Source: three-view drawing plus pictorial views. Frame: mm from the lowest corner of the part. A direction names the side the tool comes from. Give positions to 0.01 mm unless a question says otherwise; leave off trailing zeros. Write each loop counter-clockwise with the first axis right and the second up, starting at its lowest first coordinate (ties: lowest second). Pieces come first, ordered by that corner, then holes.
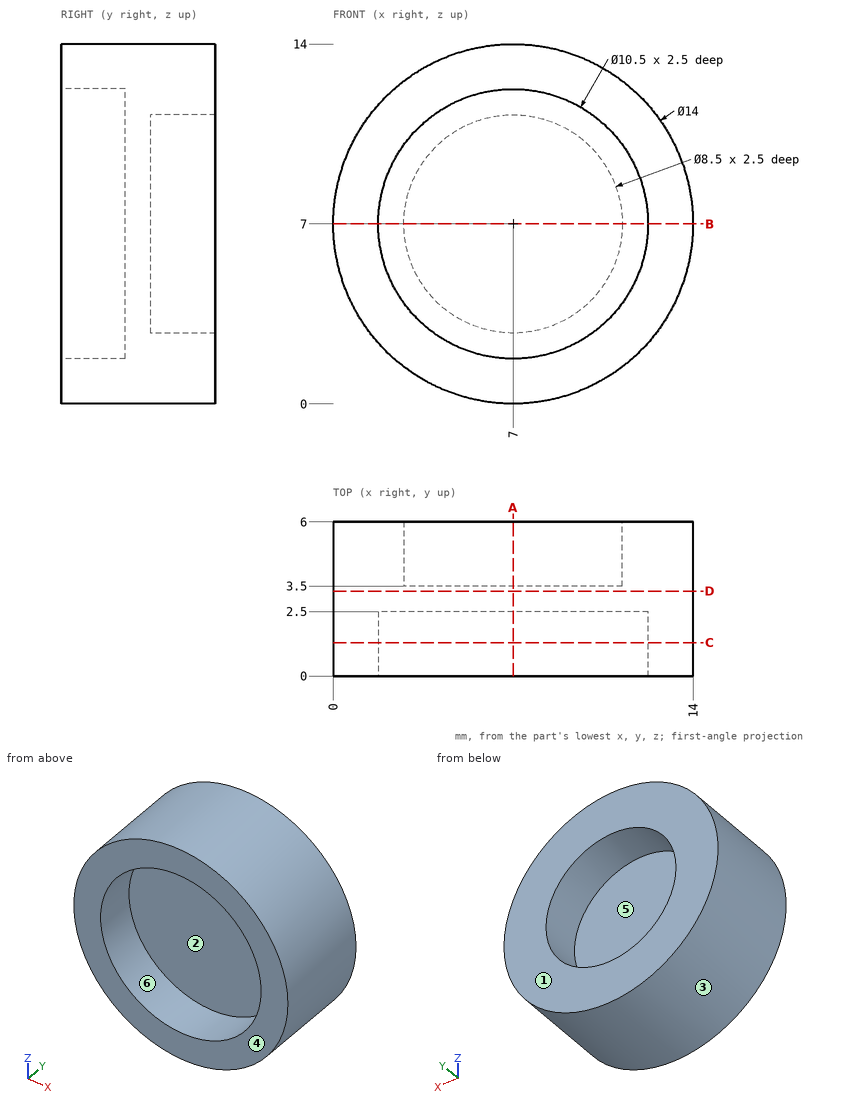
Q1. Section C-C on y = 1.3. Output: boundary loops of the cut face in (x, z).
Filled sheet:
outline: circle Ø14 at (7, 7); hole circle Ø10.5 at (7, 7)
Q2. Section B-B on z = 7. Output: boundary loops of the cut face in (x, y).
Filled sheet:
outline: (0, 0) - (1.75, 0) - (1.75, 2.5) - (12.25, 2.5) - (12.25, 0) - (14, 0) - (14, 6) - (11.25, 6) - (11.25, 3.5) - (2.75, 3.5) - (2.75, 6) - (0, 6) - close
Q3. Pull-direction query (X, two-part tool) for the marked faces 1, 2 and 3; classes: released by +X, released by -X, zero draft, split by the parting line, or undercut.
Filled sheet:
face 1: zero draft
face 2: undercut
face 3: split by the parting line
Q4. Access query for the marked faces 4, 5 and 6. Directions: +Z, -Z, +X, -X, +Y, -Y. A direction counts if a zero-diameter tool reaches every point of the face in a straight line with its end or side. Return the directions, or none.
Filled sheet:
face 4: +Z, -Z, +X, -X, -Y
face 5: +Y
face 6: -Y
Q5. Pin query (flat end, axial travel): P1, Ø1, axis at y = 1, z = 11.5, coming from the +X side; P2, Ø3, axis at x = 3.5, y = 3, coming from the -Z side; P3, Ø3, axis at x = 3.5, y = 5, coming from the +Z side; P4, Ø4, axis at x = 3.5, z = 3, coming from the -Y side. Return the tip coordinate at first contact, or that it passes through.
Filled sheet:
P1: stops at x = 12.74
P2: stops at z = 0.29
P3: stops at z = 13.71
P4: stops at y = 0
Q6. Ray query, line 1 along Z through (x, y) = (7, 0.7); line 2 along X through (y, z) = (5.4, 7). Return the intervals inside material, ascending.
Filled sheet:
line 1: z = 0 to 1.75, 12.25 to 14
line 2: x = 0 to 2.75, 11.25 to 14
Q7. Section D-D on y = 3.3. Output: boundary loops of the cut face in (x, z), plus the area to 3 significant figures.
Filled sheet:
outline: circle Ø14 at (7, 7)
area: 154 mm2
Q8. Section A-A on x = 7. Output: boundary loops of the cut face in (y, z).
Filled sheet:
outline: (0, 0) - (6, 0) - (6, 2.75) - (3.5, 2.75) - (3.5, 11.25) - (6, 11.25) - (6, 14) - (0, 14) - (0, 12.25) - (2.5, 12.25) - (2.5, 1.75) - (0, 1.75) - close
